For this review, take the finished solid that the model builds, in its own axes (mm). Round coordinates to 2 decimals unless told otherwise and drop trailing zeros. Order: outer loops, then holes, each group sorted by start corner. A loop starts at its lowest first (then second) coordinate and runs counter-clockwise, first axis right, second up. Notation, with made-up numbers: (39.5, -8.5) - (85.5, -8.5) arc R32 ccw to (85.5, 25.5) - close; hole circle Ø4 at (74, 7.5). An arc over 180 degrees is marked (long way). One line per question, with ' | ' between items.
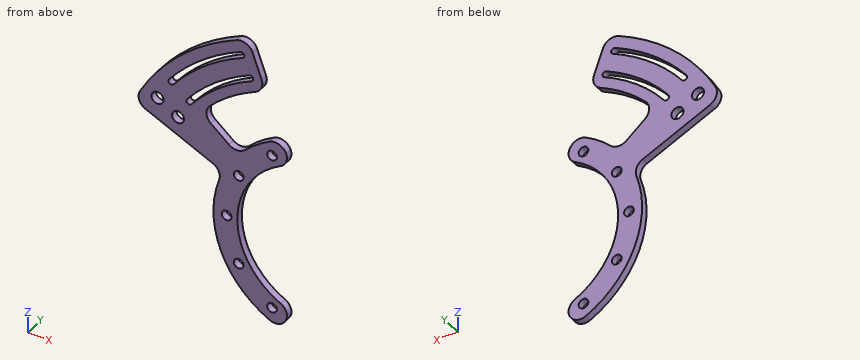
```python
from build123d import *

# Parameters (mm, degrees)
SKETCH1_R               = 43.5
SKETCH1_R_2             = 33.5
BOSS_EXTRUDE1_DEPTH     = 3
SKETCH3_R               = 2.025
CUT_EXTRUDE2_DEPTH      = 62.591395503
CIRPATTERN1_COUNT       = 12
CUT_EXTRUDE1_DEPTH      = 62.591395503
BOSS_EXTRUDE2_DEPTH     = 3
CUT_EXTRUDE_THIN1_DEPTH = 3
FILLET1_R               = 1.2
FILLET2_R               = 5
CUT_EXTRUDE3_DEPTH      = 108.998410492
CUT_EXTRUDE3_DEPTH_BACK = 108.998410492
SKETCH6_R               = 2.525


with BuildPart() as part:
    # Sketch1 → Boss-Extrude1 (new body)
    with BuildSketch(Plane(origin=(0, 0, 0), x_dir=(1, 0, 0), z_dir=(0, 1, 0))):
        with Locations(Location((0, 0, 0), (0, 0, 270))):
            Circle(SKETCH1_R)
        with Locations(Location((0, 0, 0), (0, 0, 270))):
            Circle(SKETCH1_R_2, mode=Mode.SUBTRACT)
    extrude(amount=BOSS_EXTRUDE1_DEPTH)

    # Sketch3 → Cut-Extrude2 (cut, symmetric)
    with BuildSketch(Plane(origin=(0, 3, 0), x_dir=(1, 0, 0), z_dir=(0, 1, 0))):
        with Locations(Location((-38, 0, 0), (0, 0, 270))):
            Circle(SKETCH3_R)
    cut_extrude2 = extrude(amount=CUT_EXTRUDE2_DEPTH, both=True, mode=Mode.SUBTRACT)

    # CirPattern1: Cut-Extrude2 ×12 about axis
    cirpattern1_axis = Axis((0, 0, 0), (0, 1, 0))
    for i in range(1, CIRPATTERN1_COUNT):
        add(cut_extrude2.rotate(cirpattern1_axis, i * 360 / CIRPATTERN1_COUNT), mode=Mode.SUBTRACT)

    # Sketch2 → Cut-Extrude1 (cut, symmetric)
    with BuildSketch(Plane(origin=(0, 3, 0), x_dir=(1, 0, 0), z_dir=(0, 1, 0))):
        with BuildLine():
            Line((0, 0), (43.5, 0))
            ThreePointArc((43.5, 0), (24.950574981, -35.633113927), (-14.877876235, -40.876629004))
            Line((-14.877876235, -40.876629004), (0, 0))
        make_face()
    cut_extrude1 = extrude(amount=CUT_EXTRUDE1_DEPTH, both=True, mode=Mode.SUBTRACT)

    # Mirror1: Cut-Extrude1 across plane
    add(cut_extrude1.mirror(Plane.XY), mode=Mode.SUBTRACT)

    # Sketch4 → Boss-Extrude2 (add)
    with BuildSketch(Plane(origin=(0, 0, 0), x_dir=(1, 0, 0), z_dir=(0, 1, 0))):
        with BuildLine():
            ThreePointArc((-33.322933276, -27.961261021), (-36.687527893, -23.372532963), (-39.424388736, -18.383894386))
            Line((-39.424388736, -18.383894386), (-57.550544477, -26.836259621))
            Line((-57.550544477, -26.836259621), (-76.583008005, -35.711243117))
            ThreePointArc((-76.583008005, -35.711243117), (-57.087372544, -62.29993496), (-28.900702111, -79.404026456))
            Line((-28.900702111, -79.404026456), (-21.718279101, -59.67048142))
            ThreePointArc((-21.718279101, -59.67048142), (-36.422103708, -52.016154812), (-48.643822138, -40.817013215))
            Line((-48.643822138, -40.817013215), (-33.322933276, -27.961261021))
        make_face()
    extrude(amount=BOSS_EXTRUDE2_DEPTH)

    # Sketch5 → Cut-Extrude-Thin1 (cut)
    with BuildSketch(Plane(origin=(0, 3, 0), x_dir=(1, 0, 0), z_dir=(0, 1, 0))):
        with BuildLine():
            ThreePointArc((-55.318354903, -43.219435568), (-42.735052316, -55.693404488), (-27.42932522, -64.619440712))
            Line((-27.42932522, -64.619440712), (-26.491570512, -62.410229064))
            ThreePointArc((-26.491570512, -62.410229064), (-41.274024887, -53.789356472), (-53.427129095, -41.741848027))
            Line((-53.427129095, -41.741848027), (-55.318354903, -43.219435568))
        make_face()
        with BuildLine():
            ThreePointArc((-62.804457062, -49.068219583), (-48.518285892, -63.230261221), (-31.141270941, -73.36423682))
            Line((-31.141270941, -73.36423682), (-30.203516232, -71.155025172))
            ThreePointArc((-30.203516232, -71.155025172), (-47.057258462, -61.326213205), (-60.913231254, -47.590632043))
            Line((-60.913231254, -47.590632043), (-62.804457062, -49.068219583))
        make_face()
    extrude(amount=-CUT_EXTRUDE_THIN1_DEPTH, mode=Mode.SUBTRACT)

    # Fillet1
    fillet1_edges = [part.edges().sort_by_distance(p)[0] for p in [
        (-55.318354903, 1.5, 43.219435568),
        (-62.804457062, 1.5, 49.068219583),
        (-53.427129095, 1.5, 41.741848027),
        (-60.913231254, 1.5, 47.590632043),
        (-26.491570512, 1.5, 62.410229064),
        (-30.203516232, 1.5, 71.155025172),
        (-27.42932522, 1.5, 64.619440712),
        (-31.141270941, 1.5, 73.36423682),
    ]]
    fillet(fillet1_edges, radius=FILLET1_R - 0.0001)  # a hair under: the kernel refuses the full size

    # Fillet2
    fillet2_edges = [part.edges().sort_by_distance(p)[0] for p in [
        (-14.877876235, 1.5, -40.876629004),
        (-11.457674801, 1.5, -31.479702796),
        (-11.457674801, 1.5, 31.479702796),
        (-14.877876235, 1.5, 40.876629004),
        (-39.424388736, 1.5, 18.383894386),
        (-76.583008005, 1.5, 35.711243117),
        (-28.900702111, 1.5, 79.404026456),
        (-21.718279101, 1.5, 59.67048142),
        (-33.322933276, 1.5, 27.961261021),
        (-48.643822138, 1.5, 40.817013215),
    ]]
    fillet(fillet2_edges, radius=FILLET2_R - 0.0001)  # a hair under: the kernel refuses the full size

    # Sketch6 → Cut-Extrude3 (cut, two sides: drawn at the far end of the back side and taken through both)
    with BuildSketch(Plane(origin=(0, 3, 0), x_dir=(1, 0, 0), z_dir=(0, 1, 0)).offset(-CUT_EXTRUDE3_DEPTH_BACK)):
        with Locations(Location((-58.287376448, -35.022589094, 0), (0, 0, 270))):
            Circle(SKETCH6_R)
        with Locations(Location((-66.859049455, -40.172969843, 0), (0, 0, 270))):
            Circle(SKETCH6_R)
    extrude(amount=CUT_EXTRUDE3_DEPTH + CUT_EXTRUDE3_DEPTH_BACK, mode=Mode.SUBTRACT)


solid = part.part
```
(1) For probe 1 along Z at (x, y) = (-37, 1.85); probe 2 along X at (y, z) = (0.75, 35.5); probe 3 along Z at (x, y) = (-57, 1.3), list the stretches that pass through material, from the lowest coordinate up. Write a range as [from, to].
Output values:
probe 1: [-22.87, -1.76], [1.76, 31.05], [51.61, 56.81], [59.66, 67.87], [70.59, 75.97] | probe 2: [-74.09, -60.77], [-55.81, -42.31], [-25.14, -12.94] | probe 3: [26.58, 32.85], [37.19, 52.21], [55.71, 62.38]
(2) We need section A-A on x = -68. State the section outline as (y, z) points, plus the area to 3 significant figures.
Output values:
outline: (0, 31.71) - (3, 31.71) - (3, 37.92) - (0, 37.92) - close; (0, 42.43) - (3, 42.43) - (3, 50.16) - (0, 50.16) - close | area: 41.8 mm^2
(3) We need section B-B on z = -19. State the section outline as (x, y) points.
Output values:
outline: (-39.13, 0) - (-34.93, 0) - (-34.93, 3) - (-39.13, 3) - close; (-30.88, 0) - (-27.59, 0) - (-27.59, 3) - (-30.88, 3) - close
(4) Insertion check: pin 1 (1 mm diameter, centred on x = -40, z = 63, fed in from -Y). The pin has a flat end and moves straight along its axis. Give the tip position at first contact, or say it passes through.
Output values:
pin 1: y = 0
(5) We need section C-C on x = -19. State the section outline as (y, z) points.
Output values:
outline: (0, -39) - (3, -39) - (3, -34.93) - (0, -34.93) - close; (0, -30.88) - (3, -30.88) - (3, -27.59) - (0, -27.59) - close; (0, 27.59) - (3, 27.59) - (3, 30.88) - (0, 30.88) - close; (0, 34.93) - (3, 34.93) - (3, 39) - (0, 39) - close
(6) We need section D-D on z = 59. State the section outline as (x, y) points.
Output values:
outline: (-60.49, 0) - (-53.58, 0) - (-53.58, 3) - (-60.49, 3) - close; (-49.94, 0) - (-38.04, 0) - (-38.04, 3) - (-49.94, 3) - close; (-33.4, 0) - (-24.48, 0) - (-24.48, 3) - (-33.4, 3) - close
